CAD build for the part. Positions are in the model's coordinates, mm. A direction names the side the tool comes from. Round coordinates to 2 decimals unless told otherwise and drop trailing zeros. Loops run counter-clockwise (first coordinate to the right, second up) from the corner with the lowest first, then second, coordinate; pieces in that order, holes last. Notation, with made-up numbers: (53.25, -16.5) - (65.25, -16.5) arc R21 cw to (65.25, -2.5) - close; hole circle Ø4 at (0, -35). An arc over 180 degrees is marked (long way). Use one line per item in the form item = value.
from build123d import *

# Parameters (mm, degrees)
SKETCH004_W    = 11.5
SKETCH004_H    = 1.25
PAD003_DEPTH   = 3
PAD_DEPTH      = 40
PAD_DEPTH_BACK = 1.6
THICKNESS_T    = -1.6
SKETCH002_R    = 1.75
PAD001_DEPTH   = 13
SKETCH003_R    = 3.5
PAD002_DEPTH   = 13
FILLET_R       = 0.6


with BuildPart() as pad003:
    # Sketch004 → Pad003 (new body)
    with BuildSketch(Plane.XZ.offset(44.6)):
        with BuildLine():
            Line((22.5, 29), (37.25, 29))
            ThreePointArc((38.25, 28), (37.957107, 28.707107), (37.25, 29))
            Line((38.25, 28), (38.25, 18))
            ThreePointArc((37.25, 17), (37.957107, 17.292893), (38.25, 18))
            Line((37.25, 17), (22.5, 17))
            ThreePointArc((21.5, 18), (21.792893, 17.292893), (22.5, 17))
            Line((21.5, 18), (21.5, 28))
            ThreePointArc((22.5, 29), (21.792893, 28.707107), (21.5, 28))
        make_face()
        with BuildLine():
            Line((-8.95, 29.8), (-3.75, 29.8))
            ThreePointArc((-2.75, 28.8), (-3.042893, 29.507107), (-3.75, 29.8))
            Line((-2.75, 28.8), (-2.75, 16.5))
            ThreePointArc((-3.75, 15.5), (-3.042893, 15.792893), (-2.75, 16.5))
            Line((-3.75, 15.5), (-8.95, 15.5))
            ThreePointArc((-9.95, 16.5), (-9.657107, 15.792893), (-8.95, 15.5))
            Line((-9.95, 16.5), (-9.95, 28.8))
            ThreePointArc((-8.95, 29.8), (-9.657107, 29.507107), (-9.95, 28.8))
        make_face()
        with BuildLine():
            Line((-37.25, 24.5), (-31.25, 24.5))
            ThreePointArc((-30.25, 23.5), (-30.542893, 24.207107), (-31.25, 24.5))
            Line((-30.25, 23.5), (-30.25, 18))
            ThreePointArc((-31.25, 17), (-30.542893, 17.292893), (-30.25, 18))
            Line((-31.25, 17), (-37.25, 17))
            ThreePointArc((-38.25, 18), (-37.957107, 17.292893), (-37.25, 17))
            Line((-38.25, 18), (-38.25, 23.5))
            ThreePointArc((-37.25, 24.5), (-37.957107, 24.207107), (-38.25, 23.5))
        make_face()
        with Locations((-20.25, 17.625)):
            Rectangle(SKETCH004_W, SKETCH004_H)
        Polygon((2.333401, 7), (2.333401, 11.006851), (3.391764, 12.4), (15.751917, 12.4), (16.833401, 10.855655), (16.833401, 7), align=None)
    extrude(amount=-PAD003_DEPTH)


with BuildPart() as fillet_body:
    # Sketch001 → Pad (new body, two sides)
    with BuildSketch(Plane.XY) as pad_sk:
        with BuildLine():
            Line((-43.85, 44.6), (43.85, 44.6))
            ThreePointArc((47.85, 40.6), (46.678427, 43.428427), (43.85, 44.6))
            Line((47.85, 40.6), (47.85, -40.6))
            ThreePointArc((43.85, -44.6), (46.678427, -43.428427), (47.85, -40.6))
            Line((43.85, -44.6), (-43.85, -44.6))
            ThreePointArc((-47.85, -40.6), (-46.678427, -43.428427), (-43.85, -44.6))
            Line((-47.85, -40.6), (-47.85, 40.6))
            ThreePointArc((-43.85, 44.6), (-46.678427, 43.428427), (-47.85, 40.6))
        make_face()
    extrude(amount=PAD_DEPTH)
    extrude(pad_sk.sketch, amount=-PAD_DEPTH_BACK)

    # Thickness
    thickness_openings = [fillet_body.faces().sort_by_distance(p)[0] for p in [
        (0, 0, 40),
    ]]
    offset(amount=THICKNESS_T, openings=thickness_openings)

    # Sketch002 → Pad001 (new body)
    with BuildSketch(Plane.XY):
        with Locations((-41.25, -36)):
            Circle(SKETCH002_R)
        with Locations((41.25, -36)):
            Circle(SKETCH002_R)
        with Locations((-41.25, 16.5)):
            Circle(SKETCH002_R)
        with Locations((41.25, 36)):
            Circle(SKETCH002_R)
    extrude(amount=PAD001_DEPTH)

    # Sketch003 → Pad002 (new body)
    with BuildSketch(Plane.XY):
        with Locations((41.25, -36)):
            Circle(SKETCH003_R)
        with Locations((41.25, 36)):
            Circle(SKETCH003_R)
        with Locations((-41.25, 16.5)):
            Circle(SKETCH003_R)
        with Locations((-41.25, -36)):
            Circle(SKETCH003_R)
    extrude(amount=PAD002_DEPTH)

    # Cut: cut Pad003
    add(pad003.part, mode=Mode.SUBTRACT)

    # Fillet
    fillet_edges = [fillet_body.edges().sort_by_distance(p)[0] for p in [
        (0, 44.6, -1.6),
        (46.678427, 43.428427, -1.6),
        (47.85, 0, -1.6),
        (46.678427, -43.428427, -1.6),
        (0, -44.6, -1.6),
        (-46.678427, -43.428427, -1.6),
        (-47.85, 0, -1.6),
        (-46.678427, 43.428427, -1.6),
    ]]
    fillet(fillet_edges, radius=FILLET_R)


solid = fillet_body.part
1) Slice it at B-B (z = 33). Write the cut outline in (x, y).
Report:
outline = (-47.85, -40.6) arc R4 ccw to (-43.85, -44.6) - (43.85, -44.6) arc R4 ccw to (47.85, -40.6) - (47.85, 40.6) arc R4 ccw to (43.85, 44.6) - (-43.85, 44.6) arc R4 ccw to (-47.85, 40.6) - close; hole (-46.25, -40.6) arc R2.4 ccw to (-43.85, -43) - (43.85, -43) arc R2.4 ccw to (46.25, -40.6) - (46.25, 40.6) arc R2.4 ccw to (43.85, 43) - (-43.85, 43) arc R2.4 ccw to (-46.25, 40.6) - close
2) Tool access for faces 4 (the flat face through (46.25, 1, 20)), 5 (the flat face through (1, -44.6, 20)): list every direction of +Z, -Z, +X, -X, +Y, -Y with a clear straight run to the whole face (end or side of a thin tool).
Report:
face_4 = +Z
face_5 = +Z, -Z, +X, -X, -Y
3) Drill centre lines: probe 1 along X at (y, z) = (18.5, 23); probe 2 along Y at (x, z) = (16, 21); probe 3 along X at (y, z) = (37.5, 5.5). Where is each one in solid material? Low to high.
Report:
probe_1 = -47.85 to -46.25, 46.25 to 47.85
probe_2 = -44.6 to -43, 43 to 44.6
probe_3 = -47.85 to -46.25, 38.09 to 44.41, 46.25 to 47.85
4) Flat gauge pins, fed straight in: pin 1 (5 mm diameter, centred on x = -31, y = 4, fed in from +Z); pin 2 (0.5 mm diameter, centred on y = -43.5, z = 24, fed in from -X); pin 3 (1.3 mm diameter, centred on y = -43.5, z = 21, fed in from +X). Where does each tip first touch, or does it go through?
Report:
pin_1 = 0
pin_2 = -46.85
pin_3 = 47.16
5) Slice it at D-D (z = 20). Write the cut outline in (x, y).
Report:
outline = (-47.85, -40.6) arc R4 ccw to (-43.85, -44.6) - (-38.25, -44.6) - (-38.25, -43) - (-43.85, -43) arc R2.4 cw to (-46.25, -40.6) - (-46.25, 40.6) arc R2.4 cw to (-43.85, 43) - (43.85, 43) arc R2.4 cw to (46.25, 40.6) - (46.25, -40.6) arc R2.4 cw to (43.85, -43) - (38.25, -43) - (38.25, -44.6) - (43.85, -44.6) arc R4 ccw to (47.85, -40.6) - (47.85, 40.6) arc R4 ccw to (43.85, 44.6) - (-43.85, 44.6) arc R4 ccw to (-47.85, 40.6) - close; (-30.25, -44.6) - (-9.95, -44.6) - (-9.95, -43) - (-30.25, -43) - close; (-2.75, -44.6) - (21.5, -44.6) - (21.5, -43) - (-2.75, -43) - close
6) Two-plate mould, pull along Y, no slides. Class faces 1 (the cylindrical face through (38.7, 38.4, 6.4)), 2 (the cylindrical face through (46.647, -43.459, 19.787)), 3 (the flat face through (-1, 44.6, 20)): +Y half, -Y half, draft (parallel to the pull), parting line (faces both ways), or undercut.
Report:
face_1 = undercut
face_2 = -Y half
face_3 = +Y half
7) Slice it at A-A (x = -16). Write the cut outline in (y, z).
Report:
outline = (-44.6, -1) arc R0.6 ccw to (-44, -1.6) - (44, -1.6) arc R0.6 ccw to (44.6, -1) - (44.6, 40) - (43, 40) - (43, 0) - (-43, 0) - (-43, 17) - (-44.6, 17) - close; (-44.6, 18.25) - (-43, 18.25) - (-43, 40) - (-44.6, 40) - close
8) Slice it at C-C (y = -1). Write the cut outline in (x, z), plus the area to 3 significant figures.
Report:
outline = (-47.85, -1) arc R0.6 ccw to (-47.25, -1.6) - (47.25, -1.6) arc R0.6 ccw to (47.85, -1) - (47.85, 40) - (46.25, 40) - (46.25, 0) - (-46.25, 0) - (-46.25, 40) - (-47.85, 40) - close
area = 281 mm^2
